```python
from build123d import *

# Parameters (mm, degrees)
SKETCH_1_R      = 70
SKETCH_1_R_2    = 3.4
EXTRUDE_1_DEPTH = 4


with BuildPart() as part:
    # Эскиз1 → Бобышка-Вытянуть1 (new body)
    with BuildSketch(Plane(origin=(0, 0, 0), x_dir=(1, 0, 0), z_dir=(0, 1, 0))):
        with Locations(Location((0, 0, 0), (0, 0, 270))):
            Circle(SKETCH_1_R)
        with Locations(Location((59, 0, 0), (0, 0, 270))):
            Circle(SKETCH_1_R_2, mode=Mode.SUBTRACT)
        with Locations(Location((41.71930009, -41.71930009, 0), (0, 0, 270))):
            Circle(SKETCH_1_R_2, mode=Mode.SUBTRACT)
        with Locations(Location((0, -59, 0), (0, 0, 270))):
            Circle(SKETCH_1_R_2, mode=Mode.SUBTRACT)
        with Locations(Location((-41.71930009, -41.71930009, 0), (0, 0, 270))):
            Circle(SKETCH_1_R_2, mode=Mode.SUBTRACT)
        with Locations(Location((-59, 0, 0), (0, 0, 270))):
            Circle(SKETCH_1_R_2, mode=Mode.SUBTRACT)
        with Locations(Location((-41.71930009, 41.71930009, 0), (0, 0, 270))):
            Circle(SKETCH_1_R_2, mode=Mode.SUBTRACT)
        with Locations(Location((0, 59, 0), (0, 0, 270))):
            Circle(SKETCH_1_R_2, mode=Mode.SUBTRACT)
        with Locations(Location((41.71930009, 41.71930009, 0), (0, 0, 270))):
            Circle(SKETCH_1_R_2, mode=Mode.SUBTRACT)
    extrude(amount=EXTRUDE_1_DEPTH)


solid = part.part
```
Design review of the part built by this model. Coordinates are the model's own, in mm. Coordinates: 2 decimals unless noted, no trailing zeros. Write each loop counter-clockwise with the first axis right and the second up, starting at its lowest first coordinate (ties: lowest second). Pieces come first, ordered by that corner, then holes. Notation, with made-up numbers: M 84.5,-8.5 L 141.5,-8.5 A24 cw 141.5,26.5 Z; hole C -39.75,16 d8. An arc over 180 degrees is marked long. Answer as a JSON object with one key per item and string values.
Item 1: Draft analysis for pull direction Z (two halves, no side actions). For faces 1 (the cylindrical face through (-42.594, 1.972, -55.55)), 2 (the cylindrical face through (38.703, 1.972, 43.288)), 3 (the flat face through (1, 4, -1)), state which applies: pulls with the +Z half, pulls with the -Z half, needs draft (parallel to the pull), parting line crosses it, or undercut.
Outcome:
{"face 1": "parting line crosses it", "face 2": "undercut", "face 3": "needs draft"}
Item 2: Insertion check: pin 1 Ø1.5 at (x, y) = (-18, 0.5) entering from +Z; pin 2 Ø1 at (x, y) = (-24, 2) entering from +Z; pin 3 Ø1.5 at (y, z) = (1.5, -45) entering from +X. Each pin has a flat end and moves straight along its axis. Give the tip position at first contact, or say it passes through.
Outcome:
{"pin 1": "z = 67.84", "pin 2": "z = 65.94", "pin 3": "x = 54.24"}
Item 3: Add section A-A, the plane x = 0. Give the boundary of the cut face in (y, z), and give its area (3 significant figures).
Outcome:
{"outline": "M 0,-70 L 4,-70 L 4,-62.4 L 0,-62.4 Z; M 0,-55.6 L 4,-55.6 L 4,55.6 L 0,55.6 Z; M 0,62.4 L 4,62.4 L 4,70 L 0,70 Z", "area": "506 mm²"}
Item 4: Add section D-D, the plane y = 2.2. State how many separate pieces and enclosed holes the cut face has, and give its area (3 significant figures).
Outcome:
{"separate pieces": "1", "enclosed holes": "8", "area": "15,100 mm²"}
Item 5: Add section C-C, the plane z = -59. Give the boundary of the cut face in (x, y).
Outcome:
{"outline": "M -37.67,0 L -3.4,0 L -3.4,4 L -37.67,4 Z; M 3.4,0 L 37.67,0 L 37.67,4 L 3.4,4 Z"}
Item 6: Add section B-B, the plane z = 0. Give the boundary of the cut face in (x, y), and give its area (3 significant figures).
Outcome:
{"outline": "M -70,0 L -62.4,0 L -62.4,4 L -70,4 Z; M -55.6,0 L 55.6,0 L 55.6,4 L -55.6,4 Z; M 62.4,0 L 70,0 L 70,4 L 62.4,4 Z", "area": "506 mm²"}
Item 7: Wall thickness on probe 1 along X at (y, z) = (2.8, 0); probe 2 along Z at (x, y) = (40, 2.4); probe 3 along X at (y, z) = (3.1, 62): over which ranges is each line inside the solid? List them lowest first.
Outcome:
{"probe 1": "-70 to -62.4, -55.6 to 55.6, 62.4 to 70", "probe 2": "-57.45 to -44.65, -38.79 to 38.79, 44.65 to 57.45", "probe 3": "-32.5 to -1.6, 1.6 to 32.5"}
